from build123d import *

# Parameters (mm, degrees)
BOSS_EXTRUDE2_DEPTH = 1


with BuildPart() as part:
    # Sketch1 → Boss-Extrude2 (new body)
    with BuildSketch(Plane(origin=(0, 0, 0), x_dir=(1, 0, 0), z_dir=(0, 1, 0))):
        with BuildLine():
            Line((0, 15), (0, 4.65))
            ThreePointArc((0, 4.65), (-0.163175848, -4.647136069), (0.326150697, 4.638547803))
            Line((0.326150697, 4.638547803), (1.052099022, 14.96305743))
            ThreePointArc((1.052099022, 14.96305743), (3.168172024, 16.491380461), (4.567296532, 14.287750081))
            ThreePointArc((4.567296532, 14.287750081), (-2.31124953, -14.82086791), (0, 15))
        make_face()
    extrude(amount=BOSS_EXTRUDE2_DEPTH)


solid = part.part
Geometry check sheet. Reference: the model listing, model coordinates, mm. A direction names the side the tool comes from. Round coordinates to 2 decimals unless told otherwise and drop trailing zeros. Loops run counter-clockwise (first coordinate to the right, second up) from the corner with the lowest first, then second, coordinate; pieces in that order, holes last.
Item 1: Thickness scan on line 1 (X direction, y = 0.7, z = 0); line 2 (X direction, y = 0.6, z = -13.5); line 3 (Z direction, x = -13.5, y = 0.2). Record the ranges inside material, lowest first.
Item 2: Cross-section at C-C on y = 0.85. Record the boundary of the cut face in (x, z), then the cut area to 3 significant figures.
Item 3: Cross-section at A-A on z = 0. Record the boundary of the cut face in (x, y), then the cut area to 3 significant figures.
Item 4: Cross-section at B-B on x = -2.25. Record the boundary of the cut face in (y, z), then the cut area to 3 significant figures.
Item 5: Mould release check, pull along X, two halves, no side actions. Record for faces 1 (the flat face through (0, 0.5, -9.9)), 2 (the cylindrical face through (-1.69, 0.493, 14.905)), 3 (the flat face through (0, 1, 6)): pulls with the +X half, pulls with the -X half, needs draft (parallel to the pull), parting line crosses it, or undercut.
Item 6: Cross-section at D-D on z = 9. Record the boundary of the cut face in (x, y).
Item 7: Access from +Z, -Z, +X, -X, +Y, -Y to the whole of each face (thin tool, end or side, straight path). Record for faces 4 (the flat face through (0, 0, 6)), 5 (the flat face through (0.684, 0.493, -9.729)).
Answer sheet:
1. line 1: x = -15 to -4.65, 4.65 to 15
1. line 2: x = -6.54 to 0, 0.95 to 6.54
1. line 3: z = -6.54 to 6.54
2. outline: (0, -15) - (0, -4.65) arc R4.65 cw (long way) to (0.33, -4.64) - (1.05, -14.96) arc R1.79 ccw (long way) to (4.57, -14.29) arc R15 ccw (long way) to start
2. area: 637 mm2
3. outline: (-15, 0) - (-4.65, 0) - (-4.65, 1) - (-15, 1) - close; (4.65, 0) - (15, 0) - (15, 1) - (4.65, 1) - close
3. area: 20.7 mm2
4. outline: (0, -14.83) - (1, -14.83) - (1, -4.07) - (0, -4.07) - close; (0, 4.07) - (1, 4.07) - (1, 14.83) - (0, 14.83) - close
4. area: 21.5 mm2
5. face 1: undercut
5. face 2: parting line crosses it
5. face 3: needs draft
6. outline: (-12, 0) - (12, 0) - (12, 1) - (-12, 1) - close
7. face 4: +Z, -Z, +X, -X, -Y
7. face 5: -Z, +Y, -Y
